Source: CAD feature listing. Evaluate the final solid. Frame: model axes, mm. A direction names the side the tool comes from. Round coordinates to 2 decimals unless told otherwise and drop trailing zeros. Write each loop counter-clockwise with the first axis right and the second up, starting at its lowest first coordinate (ties: lowest second). Pieces come first, ordered by that corner, then holes. Notation, with made-up numbers: (24, 54) - (66, 54) arc R20 ccw to (66, 91) - close; hole circle Ø5 at (70, 72). An arc over 180 degrees is marked (long way). Write item = value, one per line. Start each with the question number.
```python
from build123d import *

# Parameters (mm, degrees)
SKETCH1_R           = 1.6
SKETCH1_R_2         = 5.5
SKETCH1_W           = 20
SKETCH1_H           = 4
BOSS_EXTRUDE1_DEPTH = 3
CUT_EXTRUDE1_REACH  = 53.049
SKETCH2_R           = 1.25
CIRPATTERN1_COUNT   = 8


with BuildPart() as part:
    # Sketch1 → Boss-Extrude1 (new body)
    with BuildSketch(Plane(origin=(0, 0, 0), x_dir=(0, 0, -1), z_dir=(1, 0, 0))):
        with BuildLine():
            Line((-45.888888889, 3.899984172), (-3.111111111, 13.649944603))
            ThreePointArc((-3.111111111, 13.649944603), (14, 0), (-3.111111111, -13.649944603))
            Line((-3.111111111, -13.649944603), (-45.888888889, -3.899984172))
            ThreePointArc((-45.888888889, -3.899984172), (-49, 0), (-45.888888889, 3.899984172))
        make_face()
        with Locations((-45, 0)):
            Circle(SKETCH1_R, mode=Mode.SUBTRACT)
        Circle(SKETCH1_R_2, mode=Mode.SUBTRACT)
        with Locations((-27, 0)):
            Rectangle(SKETCH1_W, SKETCH1_H, mode=Mode.SUBTRACT)
    extrude(amount=BOSS_EXTRUDE1_DEPTH)

    # Sketch2 → Cut-Extrude1 (cut, up to next)
    with BuildSketch(Plane(origin=(3, 0, 0), x_dir=(0, 0, -1), z_dir=(1, 0, 0)), mode=Mode.PRIVATE) as cut_extrude1_sk1:
        with Locations((0, 11)):
            Circle(SKETCH2_R)
    cut_extrude1_tool1 = extrude(cut_extrude1_sk1.sketch, amount=-CUT_EXTRUDE1_REACH, mode=Mode.PRIVATE) & part.part
    cut_extrude1 = cut_extrude1_tool1.solids().sort_by_distance((3, 11, 0))[0]
    add(cut_extrude1, mode=Mode.SUBTRACT)

    # CirPattern1: Cut-Extrude1 ×8 about axis
    cirpattern1_axis = Axis((0, 0, 0), (1, 0, 0))
    for i in range(1, CIRPATTERN1_COUNT):
        add(cut_extrude1.rotate(cirpattern1_axis, i * 360 / CIRPATTERN1_COUNT), mode=Mode.SUBTRACT)


solid = part.part
```
(1) Section D-D (x = 1.7). Count the separate pieces of the cut face and the enclosed holes in it, plus the area to 3 significant figures.
(2) Contact query for a flat-ended pin moving along its axis: P1, Ø2, axis at y = -11, z = 0, coming from the +X side. Output: stop coordinate, or through.
(3) Section B-B (z = 29). Return the cut outline in (x, y), plus the area to 3 significant figures.
(4) Section A-A (y = 0). Return the cut outline in (x, z), plus the area to 3 significant figures.
(5) Section C-C (y = -11). Return the cut outline in (x, z), plus the area to 3 significant figures.
(6) Pull-direction query (Z, two-part tool) for faces 3 (the cylindrical face through (1.48, 1.08, 46.18)), 4 (the flat face through (0, -3, 10)), 5 (the flat face through (1.479, -8.843, 24.201)); classes: +Z half, -Z half, draft (parallel to the pull), parting line (faces both ways), or undercut.
(7) Ray query, L1, parallel to Y at x = 1.15, z = 0; L2, parallel to Y at x = 0.3, z = -1; L3, parallel to Z at x = 0.55, y = 0.75. Return the intervals inside material, ascending. Write a range as from..to.
(8) Reachability of faces 1 (the flat face through (3, -3, 10)), 2 (the flat face through (1, 0, 37)) from +Z, -Z, +X, -X, +Y, -Y: full face, straight path, thin tool, end or side. Return the list, or none.
Solution:
q1.separate_pieces = 1
q1.enclosed_holes = 11
q1.area = 941 mm^2
q2.P1 = through
q3.outline = (0, -7.75) - (3, -7.75) - (3, -2) - (0, -2) - close; (0, 2) - (3, 2) - (3, 7.75) - (0, 7.75) - close
q3.area = 34.5 mm^2
q4.outline = (0, -14) - (3, -14) - (3, -12.25) - (0, -12.25) - close; (0, -9.75) - (3, -9.75) - (3, -5.5) - (0, -5.5) - close; (0, 5.5) - (3, 5.5) - (3, 9.75) - (0, 9.75) - close; (0, 12.25) - (3, 12.25) - (3, 17) - (0, 17) - close; (0, 37) - (3, 37) - (3, 43.4) - (0, 43.4) - close; (0, 46.6) - (3, 46.6) - (3, 49) - (0, 49) - close
q4.area = 71.4 mm^2
q5.outline = (0, -8.66) - (3, -8.66) - (3, -1.25) - (0, -1.25) - close; (0, 1.25) - (3, 1.25) - (3, 14.74) - (0, 14.74) - close
q5.area = 62.7 mm^2
q6.face_3 = undercut
q6.face_4 = draft
q6.face_5 = +Z half
q7.L1 = -14..-12.25, -9.75..-5.5, 5.5..9.75, 12.25..14
q7.L2 = -13.96..-11.75, -10.25..-5.41, 5.41..10.25, 11.75..13.96
q7.L3 = -13.98..-12, -10..-5.45, 5.45..10, 12..17, 37..43.59, 46.41..48.93
q8.face_1 = +Z, -Z, +X, +Y, -Y
q8.face_2 = +X, -X
